Verification items for the finished model (mm, model axes). Face numbers are marked on the shaded views. A direction names the side the tool comes from. Give positions to 0.01 mm unless a question says otherwise; leave off trailing zeros. Loops run counter-clockwise (first coordinate to the right, second up) from the corner with the lowest first, then second, coordinate; pieces in that order, holes last. Notation, with made-up numbers: (33.25, 45) -> (85.25, 45) arc R7 ccw to (85.25, 55) -> close; hole circle Ø6 at (86.25, 12). An arc over 180 degrees is marked (long way). Use one line per item in the form item = value. Start each with the question number.
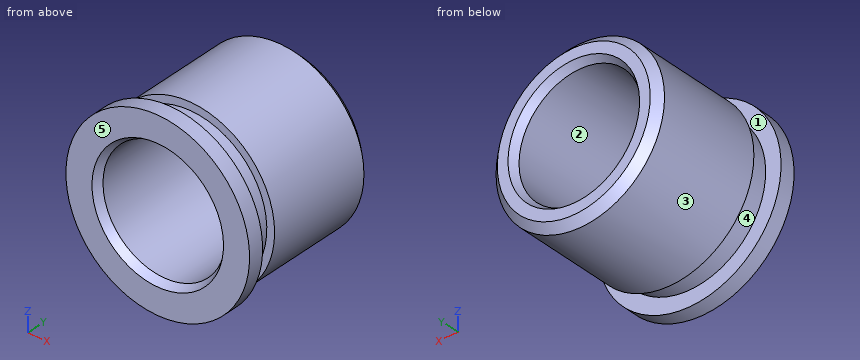
from build123d import *


with BuildPart() as part:
    # Sketch1 → Revolve1 (revolve)
    with BuildSketch(Plane.XY, mode=Mode.PRIVATE) as revolve1_sk:
        Polygon((2.146646968, -2.5019), (2.9972, -2.5019), (2.9972, -1.9939), (2.49555, -1.9939), (2.49555, -1.2319), (2.74955, -1.2319), (2.74955, 2.2479), (2.49555, 2.5019), (2.146646968, 2.5019), (2, 2.2479), (2, -2.2479), align=None)
    revolve(revolve1_sk.sketch.rotate(Axis((0, 2.5019, 0), (0, -1, 0)), 90), axis=Axis((0, 2.5019, 0), (0, -1, 0)))  # turned: the seam where the file's is


solid = part.part
Item 1: Sectioned sample at B-B, the plane z = 0. Enter the section's corners in (x, y).
Item 2: Sectioned sample at A-A, the plane x = 0. Enter the section's corners in (y, z).
Item 3: Gauge pin test, flat ends, axial feed: pin 1 Ø1.5 at (x, y) = (-1, 0) entering from +Z; pin 2 Ø1 at (x, y) = (2, -0.5) entering from -Z; pin 3 Ø1 at (y, z) = (0.5, 2) entering from -X; pin 4 Ø2.5 at (x, z) = (0, 0) entering from +Y. Record the tip position at first contact, or that the pin passes through.
Item 4: Sectioned sample at C-C, the plane y = 0.35. Enter the section's corners in (x, z).
Item 5: Draft check along Y on the marked faces 3, 4 and 5. Enter one of: +Y half, -Y half, draft (parallel to the pull), parting line (faces both ways), or undercut.
Item 6: Tool access check on the marked faces 1 and 2. Record the directions out of +Z, -Z, +X, -X, +Y, -Y that give a thin tool (end or side, any length) a straight path to the whole face; none if there is none.
Item 7: Material ranges on line 1 (X direction, y = -0.3, z = 0); line 2 (X direction, y = 0.65, z = 0.85), recorded low to high.
Outcome:
q1.outline = (-3, -2.5) -> (-2.15, -2.5) -> (-2, -2.25) -> (-2, 2.25) -> (-2.15, 2.5) -> (-2.5, 2.5) -> (-2.75, 2.25) -> (-2.75, -1.23) -> (-2.5, -1.23) -> (-2.5, -1.99) -> (-3, -1.99) -> close; (2, -2.25) -> (2.15, -2.5) -> (3, -2.5) -> (3, -1.99) -> (2.5, -1.99) -> (2.5, -1.23) -> (2.75, -1.23) -> (2.75, 2.25) -> (2.5, 2.5) -> (2.15, 2.5) -> (2, 2.25) -> close
q2.outline = (-2.5, -3) -> (-1.99, -3) -> (-1.99, -2.5) -> (-1.23, -2.5) -> (-1.23, -2.75) -> (2.25, -2.75) -> (2.5, -2.5) -> (2.5, -2.15) -> (2.25, -2) -> (-2.25, -2) -> (-2.5, -2.15) -> close; (-2.5, 2.15) -> (-2.25, 2) -> (2.25, 2) -> (2.5, 2.15) -> (2.5, 2.5) -> (2.25, 2.75) -> (-1.23, 2.75) -> (-1.23, 2.5) -> (-1.99, 2.5) -> (-1.99, 3) -> (-2.5, 3) -> close
q3.pin_1 = 2.74
q3.pin_2 = -2.3
q3.pin_3 = -2.3
q3.pin_4 = through
q4.outline = circle Ø5.5 at (0, 0); hole circle Ø4 at (0, 0)
q5.face_3 = draft
q5.face_4 = undercut
q5.face_5 = -Y half
q6.face_1 = none
q6.face_2 = +Y, -Y
q7.line_1 = -2.75 to -2, 2 to 2.75
q7.line_2 = -2.61 to -1.81, 1.81 to 2.61
